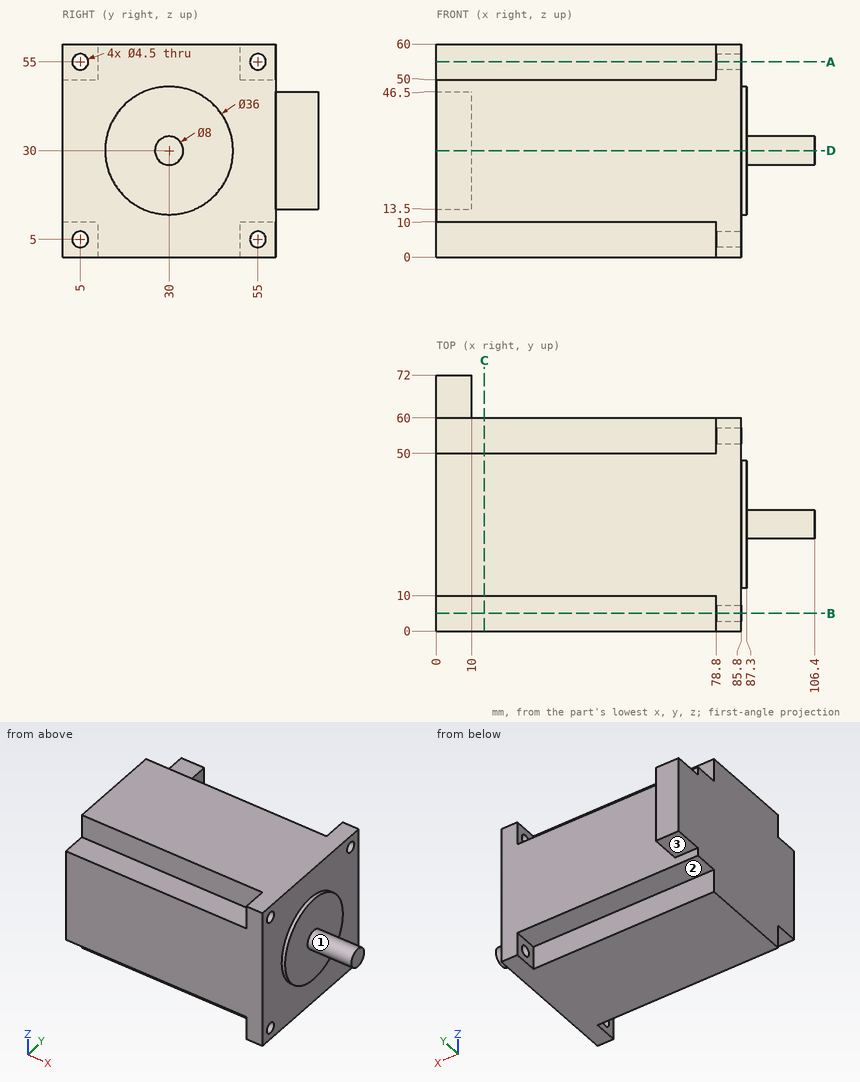
Answer from the drawing. Dimensions are ordinates in mm from the lowest x, y and z of the part. A direction names the side the tool comes from. Round coordinates to 2 decimals unless told otherwise and drop trailing zeros. Write each loop counter-clockwise with the first axis right and the second up, starting at its lowest first coordinate (ties: lowest second). Pieces come first, ordered by that corner, then holes. Notation, with made-up numbers: M 53,14 L 73,14 A30 cw 73,52 Z; hole C 24.25,78 d4. An arc over 180 degrees is marked long. One line per item, written item: value.
Q1. Straight lines are drawn through the part: line 1 (Y direction, x = 83, z = 55); line 2 (X direction, y = 14, z = 28.5); line 3 (X direction, y = 28, z = 11). For each, find the intervals that lie inside material, in ascending order. Write a range as [from, to].
Data:
line 1: [0, 2.75], [7.25, 52.75], [57.25, 60]
line 2: [0, 87.3]
line 3: [0, 85.8]
Q2. Find section A-A on z = 55. Write down the section's boundary in (x, y).
Data:
outline: M 0,10 L 78.8,10 L 78.8,7.25 L 85.8,7.25 L 85.8,52.75 L 78.8,52.75 L 78.8,50 L 0,50 Z; M 78.8,0 L 85.8,0 L 85.8,2.75 L 78.8,2.75 Z; M 78.8,57.25 L 85.8,57.25 L 85.8,60 L 78.8,60 Z
Q3. Find section D-D on z = 30. Write down the section's boundary in (x, y).
Data:
outline: M 0,0 L 85.8,0 L 85.8,12 L 87.3,12 L 87.3,26 L 106.4,26 L 106.4,34 L 87.3,34 L 87.3,48 L 85.8,48 L 85.8,60 L 10,60 L 10,72 L 0,72 Z
Q4. Find section C-C on x = 13.5. Write down the section's boundary in (y, z), plus the area to 3 significant figures.
Data:
outline: M 0,10 L 10,10 L 10,0 L 50,0 L 50,10 L 60,10 L 60,50 L 50,50 L 50,60 L 10,60 L 10,50 L 0,50 Z
area: 3,200 mm2
Q5. Which of the six approach directions +Z, -Z, +X, -X, +Y, -Y give full straight-line access (tool end or side, diameter ignored) to the marked faces 1, 2 and 3?
Data:
face 1: +X
face 2: -Z, -X, +Y
face 3: -Z, +X, -X, +Y
Q6. Flat-ended cylindrical pins translate along their axes: pin 1 Ø5 at (x, z) = (29, 3.5) entering from +Y; pin 2 Ø2.5 at (y, z) = (55, 5) entering from +X; pin 3 Ø3 at (x, y) = (34.5, 7) entering from -Z; pin 4 Ø13 at (y, z) = (68.5, 25.5) entering from +X. Find the tip coordinate at first contact, or state that the pin passes through.
Data:
pin 1: y = 50
pin 2: through
pin 3: z = 10
pin 4: x = 10
